Here's how the part is built. I have some questions about the finished solid (model axes, mm). A direction names the side the tool comes from. Give positions to 0.01 mm unless a question says otherwise; leave off trailing zeros. Write each loop counter-clockwise with the first axis right and the second up, starting at its lowest first coordinate (ties: lowest second). Pieces come first, ordered by that corner, then holes. Notation, with made-up numbers: (-39.5, -27) - (14.5, -27) arc R21 ccw to (14.5, -19) - close; hole circle Ø5 at (22, -25). An arc over 180 degrees is marked (long way). Use a Markdown table: item, result.
Autodesk Inventor part; units mm, degrees
ref_plane "YZ Plane" through (0, 0, 0) normal (1, 0, 0) x (0, 1, 0)
ref_plane "XZ Plane" through (0, 0, 0) normal (0, 1, 0) x (-1, 0, 0)
ref_plane "XY Plane" through (0, 0, 0) normal (0, 0, 1) x (1, 0, 0)
sketch "Skizze3" plane through (0, 0, 0) normal (0, 0, 1) x (1, 0, 0)
  line L0 (-500, 500) -> (500, 500)
  line L1 (500, 500) -> (500, -500)
  line L2 (500, -500) -> (-500, -500)
  line L3 (-500, -500) -> (-500, 500)
  line L4 (-500, 500) -> (-275, 500)
  line L5 (-275, 500) -> (-275, 440)
  line L6 (-275, 440) -> (-500, 440)
  line L7 (-500, 440) -> (-500, 500)
  line L8 (500, 500) -> (275, 500)
  line L9 (275, 500) -> (275, 440)
  line L10 (275, 440) -> (500, 440)
  line L11 (500, 440) -> (500, 500)
  line L12 (-275, 500) -> (275, 500)
  line L13 (275, 500) -> (275, 300)
  line L14 (275, 300) -> (-275, 300)
  line L15 (-275, 300) -> (-275, 500)
  line L16 (-225, 300) -> (225, 300)
  line L17 (225, 300) -> (225, 360)
  line L18 (225, 360) -> (-225, 360)
  line L19 (-225, 360) -> (-225, 300)
  line L20 (-500, -500) -> (500, -500)
  line L21 (500, -500) -> (500, -440)
  line L22 (500, -440) -> (-500, -440)
  line L23 (-500, -440) -> (-500, -500)
  line L24 (-440, 440) -> (-500, 440)
  line L25 (-500, 440) -> (-500, -440)
  line L26 (-500, -440) -> (-440, -440)
  line L27 (-440, -440) -> (-440, 440)
  line L28 (500, 440) -> (440, 440)
  line L29 (440, 440) -> (440, -440)
  line L30 (440, -440) -> (500, -440)
  line L31 (500, -440) -> (500, 440)
  arc A0 (-270, -10) -> (-225, 300) centre (-1315.2778, 300) ccw
  arc A1 (-500, -250) -> (-270, -10) centre (-617.8721, 93.1691) ccw
  arc A2 (225, 300) -> (280, 0) centre (1070.6818, 300) ccw
  arc A3 (280, 0) -> (500, -300) centre (931.7592, 247.2901) ccw
  arc A4 (-150, -240) -> (-95, 360) centre (-1146.8979, 153.9031) ccw
  arc A5 (-150, -240) -> (-225, -500) centre (1170.154, -761.631) ccw
  arc A6 (-5, 360) -> (105, -150) centre (4524.0164, 1069.9839) ccw
  arc A7 (125, -500) -> (105, -150) centre (-696.9412, -371.3966) ccw
  circle A8 centre (-165, 430) radius 12.5
  circle A9 centre (-65, 430) radius 12.5
  circle A10 centre (115, 430) radius 12.5
  point P0 (0, 0)
  point P1 (-500.0625, 0)
  point P2 (0, 500.0625)
  point P3 (-500, 0)
  point P4 (0, 500)
  point P5 (0, 360)
  dimension "d5" = 1000
  dimension "d8" = 1000
  dimension "d9" = 60
  dimension "d10" = 225
  dimension "d11" = 225
  dimension "d12" = 550
  dimension "d13" = 200
  dimension "d14" = 450
  dimension "d15" = 60
  dimension "d16" = 60
  dimension "d17" = 880
  dimension "d18" = 60
  dimension "d19" = 60
  dimension "d20" = 250
  dimension "d21" = 230
  dimension "d22" = 240
  dimension "d23" = 200
  dimension "d24" = 300
  dimension "d25" = 220
  dimension "d26" = 130
  dimension "d27" = 150
  dimension "d28" = 275
  dimension "d29" = 75
  dimension "d30" = 260
  dimension "d31" = 90
  dimension "d32" = 230
  dimension "d33" = 375
  dimension "d34" = 350
  dimension "d35" = 365
  dimension "d36" = 350
  dimension "d37" = 20
  dimension "d38" = 25
  dimension "d39" = 70
  dimension "d40" = 60
  dimension "d41" = 110
  dimension "d42" = 30
extrude "Extrusion2" add sketch "Skizze3" against normal blind 150 contours L0 L9 L13 L14 L17 L18 L19 L15 L5 | L19 L18 A4 L14 | L14 A6 L18 L17 | A4 L18 A6 L14 | A8 | A9 | A10
extrude "Extrusion3" cut sketch "Skizze3" against normal blind 50 contours L19 L18 A4 L14 | L14 A6 L18 L17 | A4 L18 A6 L14
extrude "Extrusion4" cut sketch "Skizze3" against normal blind 100 contours A8 | A9 | A10
equation "\"d16\" = d9"
equation "\"d18\" = d9"
equation "\"d19\" = d9"
properties part number "UA-70 Sockel"
Item 1: If we section it at C-C, the plane y = 430: Write out the boundary of the cut face in (x, z), plus the area to 3 significant figures.
Values:
| item | result |
|---|---|
| outline | (-275, -150) - (275, -150) - (275, 0) - (127.5, 0) - (127.5, -100) - (102.5, -100) - (102.5, 0) - (-52.5, 0) - (-52.5, -100) - (-77.5, -100) - (-77.5, 0) - (-152.5, 0) - (-152.5, -100) - (-177.5, -100) - (-177.5, 0) - (-275, 0) - close |
| area | 75,000 mm2 |
Item 2: I need wall thicknesses on line 1 along X through (y, z) = (333, -49); line 2 along Y through (x, z) = (-65, -60); line 3 along X through (y, z) = (437, -71.5). Which ranges of each line are inside material? Lowest first, please. Write a range as [from, to].
Values:
| item | result |
|---|---|
| line 1 | x = [-275, -225], [225, 275] |
| line 2 | y = [300, 417.5], [442.5, 500] |
| line 3 | x = [-275, -175.36], [-154.64, -75.36], [-54.64, 104.64], [125.36, 275] |
Item 3: For faces 1 (the flat face through (4, 300, -91)), 2 (the flat face through (-65, 430, -100)), 3 (the flat face through (-3, 330, -50)), which set-ups out of +Z, -Z, +X, -X, +Y, -Y let a thin tool reach every point of the face, with its end or its side?
Values:
| item | result |
|---|---|
| face 1 | +Z, -Z, +X, -X, -Y |
| face 2 | +Z |
| face 3 | +Z, -Y |
Item 4: If we section it at A-A, the plane z = -27: Write out the boundary of the cut face in (x, y).
Values:
| item | result |
|---|---|
| outline | (-275, 300) - (-225, 300) - (-225, 360) - (225, 360) - (225, 300) - (275, 300) - (275, 500) - (-275, 500) - close; hole circle Ø25 at (-165, 430); hole circle Ø25 at (-65, 430); hole circle Ø25 at (115, 430) |
Item 5: If we section it at D-D, the plane x = -194: Write out the boundary of the cut face in (y, z).
Values:
| item | result |
|---|---|
| outline | (300, -150) - (500, -150) - (500, 0) - (360, 0) - (360, -50) - (300, -50) - close |
Item 6: Thinking about a two-plate mould opening in Y: for faces 4 (the flat face through (-4, 500, -74)), 5 (the flat face through (275, 401, -74)), 6 (the cylindrical face through (-153.077, 433.755, -49.3)), which applies, +Y half, -Y half, draft (parallel to the pull), parting line (faces both ways), or undercut?
Values:
| item | result |
|---|---|
| face 4 | +Y half |
| face 5 | draft |
| face 6 | undercut |
Item 7: If we section it at B-B, the plane x = 115: Write out the boundary of the cut face in (y, z).
Values:
| item | result |
|---|---|
| outline | (300, -150) - (500, -150) - (500, 0) - (442.5, 0) - (442.5, -100) - (417.5, -100) - (417.5, 0) - (360, 0) - (360, -50) - (300, -50) - close |
Item 8: Will these pins go through, and if not, where does the flat tip stop? pin 1 Ø15 at (x, y) = (-65, 430) entering from +Z; pin 2 Ø18 at (x, y) = (-10.5, 323.5) entering from +Z; pin 3 Ø6 at (x, z) = (-136, -32) entering from -Y.
Values:
| item | result |
|---|---|
| pin 1 | stops at z = -100 |
| pin 2 | stops at z = -50 |
| pin 3 | stops at y = 360 |
